from build123d import *

# Parameters (mm, degrees)
SKETCH1_R           = 1.5
BOSS_EXTRUDE1_DEPTH = 1.6
SKETCH2_W           = 166.9
SKETCH2_H           = 96.573841314
SKETCH2_W_2         = 156.9
SKETCH2_H_2         = 86.573841314
BOSS_EXTRUDE2_DEPTH = 7.5
SKETCH3_W           = 156.9
SKETCH3_H           = 86.573841314
BOSS_EXTRUDE3_DEPTH = 4


with BuildPart() as part:
    # Sketch1 → Boss-Extrude1 (new body)
    with BuildSketch(Plane.XY):
        Polygon((-74.45, -53.48), (74.45, -53.48), (74.45, -62.135), (82.45, -62.135), (82.45, -53.48), (82.45, 53.48), (82.45, 62.135), (74.45, 62.135), (74.45, 53.48), (-74.45, 53.48), (-74.45, 62.135), (-82.45, 62.135), (-82.45, 53.48), (-82.45, -53.48), (-82.45, -62.135), (-74.45, -62.135), align=None)
        with Locations((78.45, 57.48)):
            Circle(SKETCH1_R, mode=Mode.SUBTRACT)
        with Locations((-78.45, 57.48)):
            Circle(SKETCH1_R, mode=Mode.SUBTRACT)
        with Locations(Location((-78.45, -57.48, 0), (0, 0, 180))):
            Circle(SKETCH1_R, mode=Mode.SUBTRACT)
        with Locations(Location((78.45, -57.48, 0), (0, 0, 180))):
            Circle(SKETCH1_R, mode=Mode.SUBTRACT)
    extrude(amount=BOSS_EXTRUDE1_DEPTH)

    # Sketch2 → Boss-Extrude2 (add)
    with BuildSketch(Plane(origin=(0, 0, 0), x_dir=(-1, 0, 0), z_dir=(0, 0, -1))):
        Rectangle(SKETCH2_W, SKETCH2_H)
        Rectangle(SKETCH2_W_2, SKETCH2_H_2, mode=Mode.SUBTRACT)
    extrude(amount=BOSS_EXTRUDE2_DEPTH)

    # Sketch3 → Boss-Extrude3 (add)
    with BuildSketch(Plane(origin=(0, 0, 0), x_dir=(-1, 0, 0), z_dir=(0, 0, -1))):
        Rectangle(SKETCH3_W, SKETCH3_H)
    extrude(amount=BOSS_EXTRUDE3_DEPTH)


solid = part.part
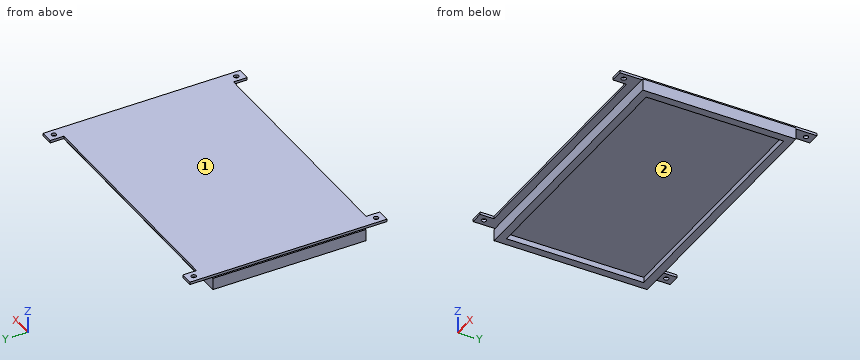
Work out the finished part from the listing and answer in its coordinate system (mm). Face numbers are marked on the shaded views. Coordinates: 2 decimals unless noted, no trailing zeros. Write each loop counter-clockwise with the first axis right and the second up, starting at its lowest first coordinate (ties: lowest second). Pieces come first, ordered by that corner, then holes. Notation, with made-up numbers: M 42,10.25 L 68,10.25 A31 cw 68,34.25 Z; hole C -27.75,61 d3. An arc over 180 degrees is marked long. Write item = value, one per line.
1. Flat-ended cylindrical pins translate along their axes: pin 1 (0.5 mm diameter, centred on y = 58, z = 0.5, fed in from -X); pin 2 (4 mm diameter, centred on x = -10.5, z = -5, fed in from -Y); pin 3 (4 mm diameter, centred on x = -40.5, y = -53, fed in from -Z); pin 4 (2.5 mm diameter, centred on x = 78.45, y = 57.48, fed in from +Z). Find the tip coordinate at first contact, or state that the pin passes through.
Solution:
pin_1 = -82.45
pin_2 = -48.29
pin_3 = 0
pin_4 = through
2. The part is cut by section C-C (x = 2). Determine the outline of the cut face in (y, z).
Solution:
outline = M -53.48,0 L -48.29,0 L -48.29,-7.5 L -43.29,-7.5 L -43.29,-4 L 43.29,-4 L 43.29,-7.5 L 48.29,-7.5 L 48.29,0 L 53.48,0 L 53.48,1.6 L -53.48,1.6 Z
3. Determine the mould class of the marked faces 1 and 2 for opening direction X: released by +X, released by -X, zero draft, split by the parting line, or undercut.
Solution:
face_1 = zero draft
face_2 = undercut
4. The part is cut by section B-B (y = 37). Determine the outline of the cut face in (x, z).
Solution:
outline = M -83.45,-7.5 L -78.45,-7.5 L -78.45,-4 L 78.45,-4 L 78.45,-7.5 L 83.45,-7.5 L 83.45,0 L 82.45,0 L 82.45,1.6 L -82.45,1.6 L -82.45,0 L -83.45,0 Z
5. Straight lines are drawn through the part: line 1 (Y direction, x = -78.45, z = 0.6) (3 decimals); line 2 (X direction, y = -57.48, z = 0.6); line 3 (Y direction, x = -6, z = -4.5). For each, find the intervals that lie inside material, in ascending order. Write a range as from..to.
Solution:
line_1 = -62.135..-58.98, -55.98..55.98, 58.98..62.135
line_2 = -82.45..-79.95, -76.95..-74.45, 74.45..76.95, 79.95..82.45
line_3 = -48.29..-43.29, 43.29..48.29
6. The part is cut by section A-A (z = -6). Determine the outline of the cut face in (x, y).
Solution:
outline = M -83.45,-48.29 L 83.45,-48.29 L 83.45,48.29 L -83.45,48.29 Z; hole M -78.45,-43.29 L 78.45,-43.29 L 78.45,43.29 L -78.45,43.29 Z
